Autodesk Inventor part; units mm, degrees
sketch "Sketch2" plane through (0, 0, 0) normal (0, 0, 1) x (1, 0, 0)
  line L0 (0, 2.8582) -> (0, -2.8582) construction
  line L1 (-5.7775, 0) -> (5.7775, 0) construction
  line L2 (0, 0) -> (4, 0)
  line L3 (4, 0) -> (-4, 0)
  circle A0 centre (0, 0) radius 4
  line L4 (0, 0) -> (-2, 3.4641)
  line L5 (0, 0) -> (4, 0) construction
  line L6 (0, 0) -> (2, 3.4641)
  line L7 (0, 0) -> (4, 0) construction
  line L8 (0, 0) -> (4, 0)
  line L9 (0, 0) -> (2, -3.4641)
  line L10 (0, 0) -> (-2, -3.4641)
  line L11 (-2, 3.4641) -> (2, 3.4641)
  line L12 (2, 3.4641) -> (4, 0)
  line L13 (4, 0) -> (2, -3.4641)
  line L14 (2, -3.4641) -> (-2, -3.4641)
  line L15 (-2, -3.4641) -> (-4, 0)
  line L16 (-4, 0) -> (-2, 3.4641)
  dimension "d3" = 4
  dimension "d2" = 8
  dimension "d1" = 120
  dimension "d0" = 60
extrude "Extrusion1" add sketch "Sketch2" along normal blind 43.5 contours L6 L12 L2 | L10 L15 L3 | L3 L16 L4 | L4 L11 L6 | L2 L13 L9 | L9 L14 L10
sketch "Sketch3" plane through (0, 0, 43.5) normal (0, 0, 1) x (1, 0, 0)
  point P0 (0, 0)
  point P1 (0, 0)
hole "Hole1" at (0, 0, 43.5) direction (0, 0, -1) diameter 4.2 depth 44
sketch "Sketch5" plane through (0, 0, 43.5) normal (0, 0, 1) x (1, 0, 0)
  line L0 (0, 0) -> (0, -56.314)
  line L1 (0, -56.314) -> (4, -56.314)
  line L2 (4, -56.314) -> (2, -59.7781)
  line L3 (2, -59.7781) -> (-2, -59.7781)
  line L4 (-2, -59.7781) -> (-4, -56.314)
  line L5 (0, -56.314) -> (-4, -56.314)
  line L6 (0, -56.314) -> (0, -52.85)
  line L7 (0, -52.85) -> (2, -52.85)
  line L8 (2, -52.85) -> (4, -56.314)
  line L9 (0, -52.85) -> (-2, -52.85)
  line L10 (-2, -52.85) -> (-4, -56.314)
  line L11 (4, 0) -> (4, -56.314)
  line L12 (-4, 0) -> (-2, -3.4641)
  line L13 (-4, 0) -> (-4, -56.314)
  line L14 (0, -56.314) -> (-44.771, -56.314)
  line L15 (-44.771, -56.314) -> (-44.771, -60.314)
  line L16 (-44.771, -56.314) -> (-44.771, -52.314)
  line L17 (-44.771, -60.314) -> (-41.307, -58.3138)
  line L18 (-44.771, -52.314) -> (-41.307, -54.3142)
  line L19 (-41.307, -54.3142) -> (-41.307, -58.3138)
  line L20 (-44.771, -60.314) -> (-48.235, -58.3138)
  line L21 (-44.771, -52.314) -> (-48.235, -54.3142)
  line L22 (-48.235, -54.3142) -> (-48.235, -58.3138)
  line L23 (-44.771, -60.314) -> (-0.654, -60.314)
  line L24 (-0.654, -60.314) -> (4, -56.314)
  line L25 (-44.771, -52.314) -> (0, -52.314)
  line L26 (-4, 0) -> (0, -3.4641)
  line L27 (-2, -3.4641) -> (2, -3.4641)
  line L28 (0, -3.4641) -> (4, 0)
  line L29 (4, -56.314) -> (4, -60.314)
  line L30 (4, -60.314) -> (-1.654, -60.314)
  point P0 (-4, -52.314)
  point P1 (-0.654, -60.314)
  dimension "d21" = 56.314
  dimension "d22" = 4
  dimension "d23" = 4
  dimension "d24" = 4
  dimension "d25" = 4
  dimension "d26" = 3.4641
  dimension "d27" = 3.464
  dimension "d28" = 2
  dimension "d29" = 2
  dimension "d30" = 44.771
  dimension "d31" = 4
  dimension "d35" = 4
  dimension "d38" = 4
  dimension "d39" = 3.464
  dimension "d40" = 4
  dimension "d41" = 3.464
  dimension "d42" = 4
  dimension "d43" = 4
  dimension "d44" = 3.464
  dimension "d45" = 3.464
extrude "Extrusion2" add sketch "Sketch5" against normal blind 43.5
sketch "Sketch6" plane through (0, 0, 43.5) normal (0, 0, 1) x (1, 0, 0)
  circle A0 centre (0, 0) radius 1.7294
  line L0 (0, 0) -> (0, -56.314)
  line L1 (0, -56.314) -> (-44.771, -56.314)
  line L2 (-4, -52.314) -> (-44.771, -52.314)
  dimension "d74" = 44.771
  dimension "d75" = 4
hole "Hole3" at (0, -56.314, 43.5) at (-44.771, -56.314, 43.5) direction (0, 0, -1) diameter 4.2 depth 44
sketch "Sketch8" plane through (0, 0, 43.5) normal (0, 0, 1) x (1, 0, 0)
  circle A0 centre (0, 0) radius 2.1
  line L0 (0, 0) -> (44.771, 0)
  line L1 (44.771, 0) -> (48.771, 0)
  line L2 (44.771, 0) -> (44.771, 3.464)
  line L3 (44.771, 3.464) -> (46.771, 3.464)
  line L4 (46.771, 3.464) -> (48.771, 0)
  line L5 (44.771, 0) -> (44.771, -3.464)
  line L6 (44.771, -3.464) -> (46.771, -3.464)
  line L7 (46.771, -3.464) -> (48.771, 0)
  line L8 (44.771, 0) -> (40.771, 0)
  line L9 (44.771, -3.464) -> (42.771, -3.464)
  line L10 (42.771, -3.464) -> (40.771, 0)
  line L11 (44.771, 3.464) -> (42.771, 3.464)
  line L12 (42.771, 3.464) -> (40.771, 0)
  line L13 (2, 3.4641) -> (-2, 3.4641)
  line L14 (2, 3.4641) -> (44.771, 3.464)
  line L15 (44.771, -3.464) -> (4, -3.464)
  line L16 (4, -60.314) -> (4, 0)
  line L17 (4, -3.464) -> (2, 3.4641)
  dimension "d62" = 44.771
  dimension "d63" = 4
  dimension "d64" = 3.464
  dimension "d65" = 2
  dimension "d66" = 3.464
  dimension "d67" = 2
  dimension "d68" = 4
  dimension "d69" = 2
  dimension "d70" = 2
extrude "Extrusion3" add sketch "Sketch8" against normal blind 43.5 contours L17 L14 L12 L0 | L0 L16 L17 | L0 L10 L15 L16 | L12 L11 L2 L0 | L0 L5 L9 L10 | L2 L3 L4 L1 | L1 L7 L6 L5
sketch "Sketch9" plane through (0, 0, 43.5) normal (0, 0, 1) x (1, 0, 0)
  line L0 (0, 0) -> (44.771, 0)
  dimension "d73" = 44.771
hole "Hole5" at (44.771, 0, 43.5) direction (0, 0, -1) diameter 4.2 depth 44
sketch "Sketch10" plane through (0, 0, 43.5) normal (0, 0, 1) x (1, 0, 0)
  line L0 (4, -3.464) -> (4, -60.314)
  line L1 (46.771, -3.464) -> (4, -3.464)
  line L2 (4, -60.314) -> (46.771, -3.464)
  line L3 (21.4983, -3.464) -> (21.4983, 3.4641)
  line L4 (2, 3.4641) -> (46.771, 3.464)
  line L5 (43.6374, -7.6291) -> (38.1012, -3.464)
  line L6 (38.1012, -3.464) -> (4, -48.7904)
  line L7 (38.1012, -3.464) -> (38.1012, -3.464)
  line L8 (38.1012, -3.464) -> (46.771, -3.464)
  line L9 (4, -48.7904) -> (4, -60.314)
  line L10 (-2, 3.4641) -> (-4, 0)
  line L11 (-48.235, -54.3142) -> (-44.771, -52.314)
  line L12 (-2, 3.4641) -> (-48.235, -54.3142)
  line L13 (-33.3199, -35.6753) -> (-27.9106, -40.0039)
  line L14 (-27.9106, -40.0039) -> (-4, -10.1236)
  line L15 (-4, -52.314) -> (-4, 0)
  line L16 (2, 3.4641) -> (-2, 3.4641)
  line L17 (-4, -10.1236) -> (-2, 3.4641)
  line L18 (-27.9106, -40.0039) -> (-37.7613, -52.314)
  line L19 (-37.7613, -52.314) -> (-48.235, -54.3142)
  point P0 (0, 0)
  dimension "d83" = 6.9281
  dimension "d84" = 6.928
  dimension "d85" = 6.928
  dimension "d86" = 90
  dimension "d87" = 90
  dimension "d88" = 90
  dimension "d89" = 90
  dimension "d90" = 90
extrude "Extrusion4" add sketch "Sketch10" against normal blind 43.5 contours L17 L15 L10 | L10 L15 L14 L13 L12 | L6 L5 L2 L0 | L1 L2 L5 | L13 L18 L19 L12
properties part number "steunstuk driehoek" material "S235"
CAD build for the part. Positions are in the model's coordinates, mm. A direction names the side the tool comes from. Round coordinates to 2 decimals unless told otherwise and drop trailing zeros. Write each loop counter-clockwise with the first axis right and the second up, starting at its lowest first coordinate (ties: lowest second). Pieces come first, ordered by that corner, then holes. Notation, with made-up numbers: M -9.75,-6 L 43.25,-6 A13 ccw 43.25,16 Z; hole C -33.75,88.25 d10. An arc over 180 degrees is marked long. Use a Markdown table: item, result. Add a question column.
1. 3-axis set-ups, long thin cutter, end or side, ignore diameter. For faces 5 (the face through (21, -3.464, 22)), 6 (the face through (47.757, -1.756, 22.054)): which of +Z, -Z, +X, -X, +Y, -Y reach the whole face in a straight line?
2. Drill centre lines: probe 1 along X at (y, z) = (-23, 3); probe 2 along Y at (x, z) = (0, 23); probe 3 along X at (y, z) = (-26.5, 21). Where is each one in solid material? Low to high.
3. Slice it at B-B on y = -13.5. Give the cut face in (x, z), then the cut area to 3 significant figures.
4. Flat gauge pins, fed straight in: P1, Ø12, axis at x = -16, z = 6.5, coming from the +Y side; P2, Ø13, axis at y = -22, z = 16.5, coming from the +X side; P3, Ø2, axis at y = -3.5, z = 36, coming from the -X side. Where does each tip first touch, or does it go through?
5. Slice it at A-A on x = 0. Give the cut face in (y, z).
6. Pull direction X, two halves, no side cores. Call faces 1 (the face through (46.82, 0.46, 21.45)), 2 (the face through (-46.479, -59.328, 22.054)), 3 (the face through (-0.092, -54.216, 21.446)), 4 (the face through (25.086, -32.287, 22.054)): released by +X, released by -X, zero draft, split by the parting line, or undercut.
7. Slice it at C-C on z = 29.5. Give the cut face in (x, y) (3 decimals).
8. Slice it at D-D on x = -11. Give the cut face in (y, z), then the cut area to 3 significant figures.
Reply:
| question | item | result |
|---|---|---|
| 1 | face 5 | +Z, -Z |
| 1 | face 6 | +Z, -Z, +X, -Y |
| 2 | probe 1 | x = -23.18 to -14.3, -4 to 4, 23.4 to 32.07 |
| 2 | probe 2 | y = -60.31 to -58.41, -54.21 to -2.1, 2.1 to 3.46 |
| 2 | probe 3 | x = -25.98 to -17.1, -4 to 4, 20.77 to 29.44 |
| 3 | outline | M -15.57,0 L -6.7,0 L -6.7,43.5 L -15.57,43.5 Z; M -4,0 L 4,0 L 4,43.5 L -4,43.5 Z; M 30.55,0 L 39.22,0 L 39.22,43.5 L 30.55,43.5 Z |
| 3 | area | 1,110 mm^2 |
| 4 | P1 | stops at y = -6.53 |
| 4 | P2 | stops at x = 37.72 |
| 4 | P3 | stops at x = -8.37 |
| 5 | outline | M -60.31,0 L -58.41,0 L -58.41,43.5 L -60.31,43.5 Z; M -54.21,0 L -2.1,0 L -2.1,43.5 L -54.21,43.5 Z; M 2.1,0 L 3.46,0 L 3.46,43.5 L 2.1,43.5 Z |
| 6 | face 1 | undercut |
| 6 | face 2 | released by -X |
| 6 | face 3 | undercut |
| 6 | face 4 | released by +X |
| 7 | outline | M -48.235,-58.314 L -44.771,-60.314 L 4,-60.314 L 46.771,-3.464 L 48.771,0 L 46.771,3.464 L 42.771,3.464 L 2,3.464 L -2,3.464 L -48.235,-54.314 Z; hole C -44.771,-56.314 d4.2; hole M -37.761,-52.314 L -4,-52.314 L -4,-10.124 Z; hole C 0,-56.314 d4.2; hole C 0,0 d4.2; hole M 4,-48.79 L 38.101,-3.464 L 4,-3.464 Z; hole C 44.771,0 d4.2 |
| 8 | outline | M -60.31,0 L -52.31,0 L -52.31,43.5 L -60.31,43.5 Z; M -18.87,0 L -7.78,0 L -7.78,43.5 L -18.87,43.5 Z |
| 8 | area | 830 mm^2 |
